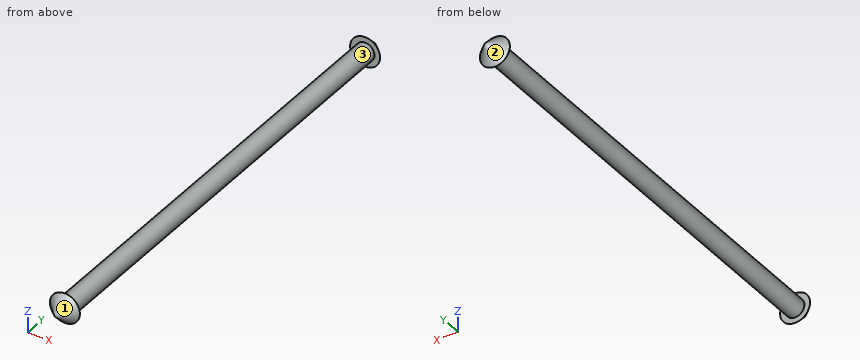
```python
from build123d import *

# Parameters (mm, degrees)
SKETCH1_R           = 2.5
BOSS_EXTRUDE1_DEPTH = 60


with BuildPart() as part:
    # Sketch1 → Boss-Extrude1 (new, symmetric)
    with BuildSketch(Plane(origin=(0, 0, 0), x_dir=(1, 0, 0), z_dir=(0, 1, 0))):
        with Locations(Location((0, 0, 0), (0, 0, 270))):
            Circle(SKETCH1_R)
    extrude(amount=BOSS_EXTRUDE1_DEPTH, both=True)


with BuildPart() as body_2:
    # Boss-Extrude2 cone 1 section (through the dimple's axis) → Boss-Extrude2 (revolve)
    with BuildSketch(Plane(origin=(0, 60, 0), x_dir=(0, 0, -1), z_dir=(1, 0, 0))):
        Polygon((0, 0), (4, 0), (0, 4), align=None)
    revolve(axis=Axis((0, 60, 0), (0, 1, 0)))


with BuildPart() as body_3:
    # Mirror1: mirrored copy
    add(body_2.part.mirror(Plane.ZX))


with BuildPart() as part_1:
    add(part.part)

    # Combine1: union body 2, body 3
    add(body_2.part)
    add(body_3.part)


solid = part_1.part
```
The model under review builds one solid part; all positions refer to its coordinate system, in mm. Face numbers are marked on the shaded views. Round coordinates to 2 decimals unless told otherwise and drop trailing zeros. Loops run counter-clockwise (first coordinate to the right, second up) from the corner with the lowest first, then second, coordinate; pieces in that order, holes last.
Item 1: Take a section at A-A (y = 29). Write out the cut boundary in (x, z), then the cut area to 3 significant figures.
Determined:
outline: circle Ø5 at (0, 0)
area: 19.6 mm2
Item 2: For line 1 (Y direction, x = -0.75, z = -2.5); line 2 (Y direction, x = 3, z = 0.5); line 3 (Z direction, x = -0.25, y = -54), list the stretches that pass through material, from the lowest coordinate up.
Determined:
line 1: y = -61.39 to -60, 60 to 61.39
line 2: y = -60.96 to -60, 60 to 60.96
line 3: z = -2.49 to 2.49
Item 3: Mouldability with a two-part tool opening along Y and no side actions: class the marked faces 1, 2 and 3 as released by +Y, released by -Y, zero draft, split by the parting line, or undercut.
Determined:
face 1: released by -Y
face 2: released by +Y
face 3: undercut
Item 4: Clearance check with flat-ended pins moving along their axes: pin 1 Ø4 at (x, y) = (-2.5, 2) entering from -Z; pin 2 Ø2 at (x, y) = (-3, -24.5) entering from -Z; pin 3 Ø1 at (y, z) = (-34, -2.5) entering from +X. State where each tip first meets the part, or that it passes through.
Determined:
pin 1: stops at z = -2.45
pin 2: stops at z = -1.5
pin 3: stops at x = 1.5
